Check sheet for the modelled part. Datum: model origin and axes. Units: mm. Face numbers are marked on the shaded views. A direction names the side the tool comes from. Round coordinates to 2 decimals unless told otherwise and drop trailing zeros. Loops run counter-clockwise (first coordinate to the right, second up) from the corner with the lowest first, then second, coordinate; pieces in that order, holes last. Notation, with made-up numbers: M -29,-34 L 21,-34 A32 cw 21,-4 Z; hole C -6.75,49.25 d4. An arc over 180 degrees is marked long. One line per question, with ' | ' between items. Start each with the question number.
(1) Tool access check on the marked faces 1 and 2. Record the directions out of +Z, -Z, +X, -X, +Y, -Y that give a thin tool (end or side, any length) a straight path to the whole face; none if there is none.
(2) Go/stop test with flat-tipped pins: P1, Ø2, axis at x = 26.5, y = 13.5, coming from the -Z side; P2, Ø0.6, axis at x = 26.5, y = 13.5, coming from the -Z side; P3, Ø12, axis at x = 17, z = -21, coming from the +Y side. Record where each tip stops, or that it passes through.
(3) Thickness scan on probe 1 along Z at (x, y) = (20.5, 7.25); probe 2 along Z at (x, y) = (7.25, 2); probe 3 along Y at (x, z) = (19, -8). Record the ranges inside material, lowest first. Write a range as [from, to].
(4) Section check A-A (x = 7.5). Record the boundary of the cut face in (y, z).
(5) Section check D-D (z = -23.5). Record the boundary of the cut face in (x, y), and give its area (3 significant figures).
(6) Section check B-B (x = 27.5). Record the boundary of the cut face in (y, z).
(7) Section check C-C (y = 2.25). Record the boundary of the cut face in (x, z).
```python
from build123d import *

# Parameters (mm, degrees)
SKETCH1_W           = 30
SKETCH1_H           = 75
BOSS_EXTRUDE1_DEPTH = 12
CUT_EXTRUDE1_DEPTH  = 12
LPATTERN1_COUNT     = 3
LPATTERN1_PITCH     = 20
BOUNDARY1_START     = -45
BOUNDARY1_DEPTH     = 5
LPATTERN2_COUNT     = 3
LPATTERN2_PITCH     = 20


# Read off the part's stored shape, not the designer's step: Boundary1
with BuildPart() as part:
    # Sketch1 → Boss-Extrude1 (new body)
    with BuildSketch(Plane(origin=(0, 0, 0), x_dir=(1, 0, 0), z_dir=(0, 1, 0))):
        with Locations((15, 37.5)):
            Rectangle(SKETCH1_W, SKETCH1_H)
    extrude(amount=BOSS_EXTRUDE1_DEPTH)

    # Sketch3 → Cut-Extrude1 (cut)
    with BuildSketch(Plane(origin=(0, 0, 0), x_dir=(1, 0, 0), z_dir=(0, 1, 0))):
        Polygon((0, 5), (22.5, 12.5), (0, 20), align=None)
    cut_extrude1 = extrude(amount=CUT_EXTRUDE1_DEPTH, mode=Mode.SUBTRACT)

    # LPattern1: Cut-Extrude1 ×3
    with Locations(*[(0, 0, -i * LPATTERN1_PITCH) for i in range(1, LPATTERN1_COUNT)]):
        add(cut_extrude1, mode=Mode.SUBTRACT)

    # Boundary1 outline → Boundary1 (add)
    with BuildSketch(Plane.XY.offset(BOUNDARY1_START)):
        Polygon((30, 14), (25, 12), (30, 12), align=None)
    boundary1 = extrude(amount=BOUNDARY1_DEPTH)

    # LPattern2: Boundary1 ×3
    with Locations(*[(0, 0, i * LPATTERN2_PITCH) for i in range(1, LPATTERN2_COUNT)]):
        add(boundary1)


solid = part.part
```
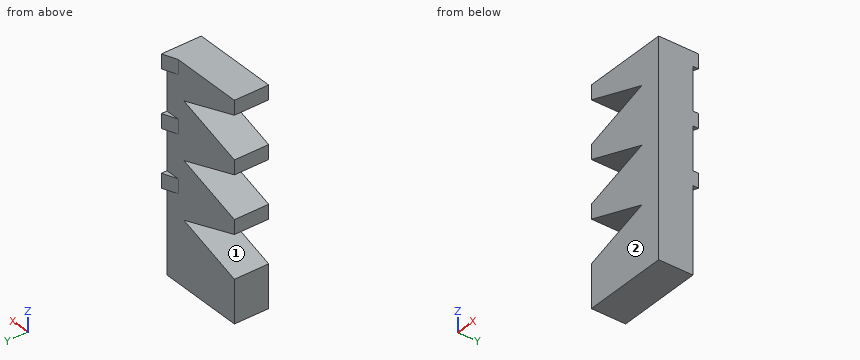
The answers:
1) face 1: -X, +Y, -Y | face 2: +Z, -Z, +X, -X, -Y
2) P1: z = -45 | P2: through | P3: y = 12
3) probe 1: [-75, -53.17], [-51.83, -33.17], [-31.83, -13.17], [-11.83, 0] | probe 2: [-75, -57.58], [-47.42, -37.58], [-27.42, -17.58], [-7.42, 0] | probe 3: [0, 12]
4) outline: M 0,-75 L 12,-75 L 12,-57.5 L 0,-57.5 Z; M 0,-47.5 L 12,-47.5 L 12,-37.5 L 0,-37.5 Z; M 0,-27.5 L 12,-27.5 L 12,-17.5 L 0,-17.5 Z; M 0,-7.5 L 12,-7.5 L 12,0 L 0,0 Z
5) outline: M 0,0 L 30,0 L 30,14 L 25,12 L 0,12 Z | area: 365 mm²
6) outline: M 0,-75 L 12,-75 L 12,-45 L 13,-45 L 13,-40 L 12,-40 L 12,-25 L 13,-25 L 13,-20 L 12,-20 L 12,-5 L 13,-5 L 13,0 L 0,0 Z
7) outline: M 0,-75 L 30,-75 L 30,0 L 0,0 L 0,-5 L 22.5,-12.5 L 0,-20 L 0,-25 L 22.5,-32.5 L 0,-40 L 0,-45 L 22.5,-52.5 L 0,-60 Z
